Could you check a few things on this model? Use its own coordinates, in mm. A direction names the side the tool comes from. Coordinates: 2 decimals unless noted, no trailing zeros. Loops run counter-clockwise (first coordinate to the right, second up) from the corner with the lowest first, then second, coordinate; pieces in that order, holes last.
1) Imagine slicing it at D-D on y = -11. Please give me the cut outline in (x, z), plus the area to 3 significant figures.
2) Imagine slicing it at A-A on y = -20. Please give me the cut outline in (x, z), plus the area to 3 significant figures.
3) Thinking about a two-plate mould opening in X: for faces 1 (the face through (20.89, 21.01, 8.87)), 2 (the face through (0, 25, 9)), 3 (the face through (20.89, -18.99, 8.87)), 4 (the face through (-25, -11, 9)), which applies, released by +X, released by -X, zero draft, split by the parting line, or undercut?
4) Imagine slicing it at C-C on x = -22. Please give me the cut outline in (y, z), plus the area to 3 significant figures.
5) If I drill on line 1 along Y through (x, z) = (-22, 12.5); line 2 along Y through (x, z) = (-26.5, 16.25); line 3 along X through (y, z) = (-3.5, 3), over which ranges is the centre line in solid material (lowest first)?
6) Will these pins go through, and if not, where does the flat tip stop? P1, Ø9.5, axis at y = 22.5, z = 8.5, coming from the -X side; P2, Ø7, axis at x = -29.5, z = 6.5, coming from the +Y side; P3, Ø7, axis at x = -34.5, z = 10, coming from the -Y side.
7) For faces 5 (the face through (-38.86, 10, 9)), 6 (the face through (-32, 3.899, 9)), 7 (the face through (-25, 21, 9)), which set-ups out of +Z, -Z, +X, -X, +Y, -Y let a thin tool reach every point of the face, with its end or its side?
8) Imagine slicing it at B-B on z = 14.5. Please give me the cut outline in (x, y).
```python
from build123d import *

# Parameters (mm, degrees)
SKETCH_1_W      = 50
SKETCH_1_H      = 50
SKETCH_1_R      = 1.5
EXTRUDE_1_DEPTH = 18
SKETCH_2_W      = 13.860098184
SKETCH_2_H      = 12.505152703
EXTRUDE_2_DEPTH = 18


with BuildPart() as part:
    # 草图1 → 凸台-拉伸1 (new body)
    with BuildSketch(Plane.XY):
        Rectangle(SKETCH_1_W, SKETCH_1_H)
        with Locations((-22, 20)):
            Circle(SKETCH_1_R, mode=Mode.SUBTRACT)
        with Locations((-22, -20)):
            Circle(SKETCH_1_R, mode=Mode.SUBTRACT)
        with Locations((22, 20)):
            Circle(SKETCH_1_R, mode=Mode.SUBTRACT)
        with Locations((22, -20)):
            Circle(SKETCH_1_R, mode=Mode.SUBTRACT)
    extrude(amount=EXTRUDE_1_DEPTH)

    # 草图2 → 凸台-拉伸2 (add)
    with BuildSketch(Plane.XY.offset(18)):
        with Locations((-31.930049092, 10.152032571)):
            Rectangle(SKETCH_2_W, SKETCH_2_H)
    extrude(amount=-EXTRUDE_2_DEPTH)


solid = part.part
```
Filled in:
1. outline: (-25, 0) - (25, 0) - (25, 18) - (-25, 18) - close
1. area: 900 mm2
2. outline: (-25, 0) - (-23.5, 0) - (-23.5, 18) - (-25, 18) - close; (-20.5, 0) - (20.5, 0) - (20.5, 18) - (-20.5, 18) - close; (23.5, 0) - (25, 0) - (25, 18) - (23.5, 18) - close
2. area: 792 mm2
3. face 1: undercut
3. face 2: zero draft
3. face 3: undercut
3. face 4: released by -X
4. outline: (-25, 0) - (-21.5, 0) - (-21.5, 18) - (-25, 18) - close; (-18.5, 0) - (18.5, 0) - (18.5, 18) - (-18.5, 18) - close; (21.5, 0) - (25, 0) - (25, 18) - (21.5, 18) - close
4. area: 792 mm2
5. line 1: y = -25 to -21.5, -18.5 to 18.5, 21.5 to 25
5. line 2: y = 3.9 to 16.4
5. line 3: x = -25 to 25
6. P1: stops at x = -25
6. P2: stops at y = 16.4
6. P3: stops at y = 3.9
7. face 5: +Z, -Z, -X, +Y, -Y
7. face 6: +Z, -Z, -X, -Y
7. face 7: +Z, -Z, -X, +Y
8. outline: (-38.86, 3.9) - (-25, 3.9) - (-25, -25) - (25, -25) - (25, 25) - (-25, 25) - (-25, 16.4) - (-38.86, 16.4) - close; hole circle Ø3 at (-22, -20); hole circle Ø3 at (-22, 20); hole circle Ø3 at (22, -20); hole circle Ø3 at (22, 20)
